The listing builds one solid part. Answer for the finished solid, in the listing's coordinates (mm). A direction names the side the tool comes from. Round coordinates to 2 decimals unless told otherwise and drop trailing zeros. Write each loop counter-clockwise with the first axis right and the second up, starting at its lowest first coordinate (ties: lowest second). Pieces come first, ordered by that corner, then holes. Notation, with made-up numbers: M 65.5,36 L 90.5,36 A35 cw 90.5,75 Z; hole C 68.5,7 d9. An arc over 180 degrees is marked long. Put each result on its own line as item: value. Start each with the question number.
```python
from build123d import *

# Parameters (mm, degrees)
F1_DEPTH = 184
F2_W     = 50
F2_H     = 65
F3_DEPTH = 321
F4_R     = 10


with BuildPart() as f1:
    # F0 (on Front) → F1 (new body)
    with BuildSketch(Plane.XZ):
        with BuildLine():
            Line((0, 157.123631), (0, 0))
            Line((0, 0), (108.799577, 0))
            Line((108.799577, 0), (108.799577, 83.561815))
            Line((108.799577, 83.561815), (59.399788, 167.123631))
            Line((59.399788, 167.123631), (10, 167.123631))
            ThreePointArc((10, 167.123631), (2.928932, 164.194698), (0, 157.123631))
        make_face()
    extrude(amount=F1_DEPTH)

    # F2 (on face) → F3 (cut)
    with BuildSketch(Plane.XZ.offset(184)):
        with Locations((83.799577, 32.5)):
            Rectangle(F2_W, F2_H)
    extrude(amount=-F3_DEPTH, mode=Mode.SUBTRACT)

    # F4
    f4_edges = [f1.edges().sort_by_distance(p)[0] for p in [
        (58.799577, -92, 65),
    ]]
    fillet(f4_edges, radius=F4_R)


solid = f1.part
```
Item 1: Flat-ended cylindrical pins translate along their axes: pin 1 (16.5 mm diameter, centred on y = -131.5, z = 16.5, fed in from +X); pin 2 (2 mm diameter, centred on y = -126, z = 123.5, fed in from +X). Find the tip coordinate at first contact, or state that the pin passes through.
Item 2: Consider line 1 along X through (y, z) = (-42, 7.5); line 2 along Z through (x, y) = (7, -113.5); line 3 along X through (y, z) = (-101, 159.5). Determine where each line is inside the solid, lowest interval first. Write a range as [from, to].
Item 3: Which of the six approach directions +Z, -Z, +X, -X, +Y, -Y give full straight-line access (tool end or side, diameter ignored) to faces 1 (the flat face through (58.8, -93, 27)), 2 (the cylindrical face through (3.007, -90.712, 164.272))?
Item 4: Section A-A (y = -122.5) is taken. Give the vertices of the cut face in (x, z).
Item 5: Section B-B (z = 52) is taken. Give the vertices of the cut face in (x, y).
Item 6: Section C-C (x = 63) is taken. Give the vertices of the cut face in (y, z).
Output values:
1. pin 1: stops at x = 58.8
1. pin 2: stops at x = 85.78
2. line 1: x = [0, 58.8]
2. line 2: z = [0, 166.66]
2. line 3: x = [0.29, 63.91]
3. face 1: -Z, +X, +Y, -Y
3. face 2: +Z, -X, +Y, -Y
4. outline: M 0,0 L 58.8,0 L 58.8,55 A10 cw 68.8,65 L 108.8,65 L 108.8,83.56 L 59.4,167.12 L 10,167.12 A10 ccw 0,157.12 Z
5. outline: M 0,-184 L 58.8,-184 L 58.8,0 L 0,0 Z
6. outline: M -184,63.15 L 0,63.15 L 0,161.03 L -184,161.03 Z
